Autodesk Inventor part; units mm, degrees
ref_plane "YZ Plane" through (0, 0, 0) normal (1, 0, 0) x (0, 1, 0)
ref_plane "XZ Plane" through (0, 0, 0) normal (0, 1, 0) x (-1, 0, 0)
ref_plane "XY Plane" through (0, 0, 0) normal (0, 0, 1) x (1, 0, 0)
sketch "Sketch1" plane through (0, 0, 0) normal (0, 1, 0) x (-1, 0, 0)
  line L0 (101.6, 101.6) -> (-101.6, 101.6)
  line L1 (-101.6, 101.6) -> (-101.6, -101.6)
  line L2 (-101.6, -101.6) -> (101.6, -101.6)
  line L3 (101.6, -101.6) -> (101.6, 101.6)
  circle A0 centre (0, 0) radius 2.5
  line L4 (9.525, -6.5) -> (-9.525, -6.5)
  line L5 (0, 0) -> (0, 8)
  line L6 (-14.5, -6.5) -> (-14.5, 22.5)
  line L7 (14.5, 22.5) -> (14.5, -6.5)
  circle A1 centre (0, 8) radius 14
  line L8 (-14.5, 22.5) -> (14.5, 22.5)
  line L9 (14.5, -6.5) -> (-14.5, -6.5)
  line L10 (-24.5, 32.5) -> (24.5, 32.5)
  line L11 (24.5, 32.5) -> (24.5, -16.5)
  line L12 (24.5, -16.5) -> (-24.5, -16.5)
  line L13 (-24.5, -16.5) -> (-24.5, 32.5)
  line L14 (-9.525, 22.5) -> (9.525, 22.5)
  line L15 (9.525, 22.5) -> (9.525, 27.58)
  line L16 (9.525, 27.58) -> (-9.525, 27.58)
  line L17 (-9.525, 27.58) -> (-9.525, 22.5)
  point P0 (9.525, 22.5)
  point P1 (-9.525, -6.5)
  dimension "d0" = 203.2
  dimension "d1" = 203.2
  dimension "d2" = 8
  dimension "d3" = 28
  dimension "d4" = 29
  dimension "d5" = 29
  dimension "d6" = 14.5
  dimension "d7" = 10
  dimension "d8" = 10
  dimension "d9" = 10
  dimension "d10" = 10
  dimension "d11" = 5.08
  dimension "d12" = 9.525
  dimension "d13" = 9.525
  dimension "d14" = 101.6
  dimension "d15" = 101.6
extrude "Extrusion1" add sketch "Sketch1" along normal blind 56.5 contours A0 | L4 L9 L6 L8 L7 | L8 L17 L16 L15 | A1 | L10 L11 L12 L13
sketch "Sketch2" plane through (0, 56.5, 0) normal (0, 1, 0) x (1, 0, 0)
  line L0 (101.6, 101.6) -> (-101.6, 101.6)
  line L1 (-101.6, 101.6) -> (-101.6, -101.6)
  line L2 (-101.6, -101.6) -> (101.6, -101.6)
  line L3 (101.6, -101.6) -> (101.6, 101.6)
  circle A0 centre (0, 0) radius 2.5
  line L4 (-9.525, 6.5) -> (9.525, 6.5)
  line L5 (0, 0) -> (0, -8)
  line L6 (14.5, 6.5) -> (14.5, -22.5)
  line L7 (-14.5, -22.5) -> (-14.5, 6.5)
  circle A1 centre (0, -8) radius 14
  line L8 (14.5, -22.5) -> (-14.5, -22.5)
  line L9 (-14.5, 6.5) -> (14.5, 6.5)
  line L10 (24.5, -32.5) -> (-24.5, -32.5)
  line L11 (-24.5, -32.5) -> (-24.5, 16.5)
  line L12 (-24.5, 16.5) -> (24.5, 16.5)
  line L13 (24.5, 16.5) -> (24.5, -32.5)
  line L14 (9.525, -22.5) -> (-9.525, -22.5)
  line L15 (-9.525, -22.5) -> (-9.525, -27.58)
  line L16 (-9.525, -27.58) -> (9.525, -27.58)
  line L17 (9.525, -27.58) -> (9.525, -22.5)
  point P0 (9.525, 22.5)
  point P1 (-9.525, -6.5)
  dimension "d18" = 203.2
  dimension "d19" = 203.2
  dimension "d20" = 8
  dimension "d21" = 28
  dimension "d22" = 29
  dimension "d23" = 29
  dimension "d24" = 14.5
  dimension "d25" = 10
  dimension "d26" = 10
  dimension "d27" = 10
  dimension "d28" = 10
  dimension "d29" = 5.08
  dimension "d30" = 9.525
  dimension "d31" = 9.525
  dimension "d32" = 101.6
  dimension "d33" = 101.6
extrude "Extrusion2" cut sketch "Sketch2" against normal blind 19.5 contours A0 | L4 L9 L6 L8 L7 | L8 L17 L16 L15 | A1
sketch "Sketch4" plane through (0, 56.5, 0) normal (0, 1, 0) x (1, 0, 0)
  circle A0 centre (-17.508, -8) radius 2
  circle A1 centre (17.4854, -8) radius 2
  circle A2 centre (17.4854, -8) radius 2
  circle A3 centre (0, -8.01) radius 14
  circle A4 centre (0, -0.01) radius 2.5
  circle A5 centre (-19.4934, 12.0285) radius 2.2448
  circle A6 centre (19.5, 12.0285) radius 2.3104
  circle A7 centre (19.5, -28.5182) radius 2.2008
  circle A8 centre (-19.4934, -28.5182) radius 2.3894
  point P0 (0, 0)
  dimension "d37" = 34.9934
  dimension "d38" = 28
  dimension "d39" = 8
  dimension "d65" = 8
  dimension "d66" = 8
hole "Hole1" at (-17.508, 56.5, 8) at (17.4854, 56.5, 8) at (-19.4934, 56.5, 28.5182) at (19.5, 56.5, 28.5182) at (-19.4934, 56.5, -12.0285) at (19.5, 56.5, -12.0285) direction (0, -1, 0) diameter 2.85 depth 12.7 tip angle 118 countersink diameter 3.0226 countersink angle 82
sketch "Sketch5" plane through (0, 0, 0) normal (0, -1, 0) x (1, 0, 0)
  circle A0 centre (-19.4934, 28.5182) radius 1.425
  circle A1 centre (-19.4934, 28.5182) radius 1.425
  circle A2 centre (19.5, 28.5182) radius 1.425
  circle A3 centre (19.5, 28.5182) radius 1.425
  circle A4 centre (19.5, -12.0285) radius 1.425
  circle A5 centre (19.5, -12.0285) radius 1.425
  circle A6 centre (-19.4934, -12.0285) radius 1.5113
  circle A7 centre (-19.4934, -12.0285) radius 1.5113
  point P0 (0, 0)
hole "Hole2" at (19.5, 0, -12.0285) at (-19.4934, 0, -12.0285) at (-19.4934, 0, 28.5182) at (19.5, 0, 28.5182) direction (0, 1, 0) diameter 2.85 depth 12.7 tip angle 118 countersink diameter 3.0226 countersink angle 82
sketch "Sketch6" plane through (-24.5, 0, 32.5) normal (0, 0, 1) x (1, 0, 0)
  line L0 (34.025, 56.5) -> (34.025, 37)
  line L1 (14.975, 56.5) -> (34.025, 56.5)
  line L2 (34.025, 56.5) -> (34.025, 46.75)
  line L3 (34.025, 46.75) -> (14.975, 46.75)
  line L4 (14.975, 46.75) -> (14.975, 56.5)
  point P0 (24.5, 0)
extrude "Extrusion3" cut sketch "Sketch6" against normal blind 25.4
sketch "Sketch8" plane through (0, 56.5, 0) normal (0, 1, 0) x (1, 0, 0)
  line L0 (-24.5, -3) -> (24.5, -3)
  line L1 (24.5, -3) -> (24.5, -13)
  line L2 (24.5, -13) -> (-24.5, -13)
  line L3 (-24.5, -13) -> (-24.5, -3)
  line L4 (14.5, 6.5) -> (14.5, -22.5)
  line L5 (14.5, -3) -> (14.5, -13)
  line L6 (-14.5, -22.5) -> (-14.5, 6.5)
  line L7 (-14.5, -3) -> (-14.5, -13)
  line L8 (24.5, -32.5) -> (24.5, 16.5)
  line L9 (-24.5, 16.5) -> (-24.5, -32.5)
  point P0 (0, 0)
  dimension "d58" = 10
  dimension "d60" = 0
  dimension "d61" = 0
  dimension "d62" = 3
extrude "Extrusion4" cut sketch "Sketch8" against normal blind 2 contours L0 L6 L2 L3 | L0 L1 L2 L4
sketch "Sketch9" plane through (0, 56.5, 0) normal (0, 1, 0) x (1, 0, 0)
  line L0 (-14.5, 6.5) -> (14.5, 6.5)
  line L1 (24.5, 16.5) -> (-24.5, 16.5)
  line L2 (-14.5, 6.5) -> (14.5, 6.5)
  line L3 (14.5, 6.5) -> (14.5, 16.5)
  line L4 (14.5, 16.5) -> (-14.5, 16.5)
  line L5 (-14.5, 16.5) -> (-14.5, 6.5)
  line L6 (14.5, 6.5) -> (14.5, -3)
  line L7 (-14.5, 11.5) -> (14.5, 11.5)
  line L8 (-24.5, 16.5) -> (-24.5, -32.5)
  line L9 (-14.5, 6.5) -> (-24.5, 6.5)
  line L10 (-24.5, 6.5) -> (-24.5, -22.5)
  line L11 (-24.5, -22.5) -> (-14.5, -22.5)
  line L12 (-14.5, -22.5) -> (-14.5, 6.5)
  line L13 (-9.525, -22.5) -> (-14.5, -22.5)
  line L14 (-20.5, 6.5) -> (-20.5, -22.5)
  line L15 (24.5, -32.5) -> (24.5, 16.5)
  line L16 (24.5, -22.5) -> (20.5, -22.5)
  line L17 (20.5, -22.5) -> (20.5, 6.5)
  line L18 (20.5, 6.5) -> (24.5, 6.5)
  line L19 (24.5, 6.5) -> (24.5, -22.5)
  point P0 (0, 0)
  point P1 (-14.5, 16.5)
  dimension "d67" = 0
  dimension "d68" = 5
  dimension "d69" = 0
  dimension "d71" = 4
  dimension "d72" = 4
extrude "Extrusion5" cut sketch "Sketch9" against normal through all contours L15 L16 L17 L18 | L5 L1 L3 L7 | L14 L11 L8 L9
sketch "Sketch11" plane through (0, 37, 0) normal (0, 1, 0) x (1, 0, 0)
  line L0 (-20.5, -3) -> (-14.5, -3)
  line L1 (20.5, -13) -> (20.5, -3)
  line L2 (-20.5, -3) -> (20.5, -3)
  line L3 (20.5, -3) -> (20.5, -13)
  line L4 (20.5, -13) -> (-20.5, -13)
  line L5 (-20.5, -13) -> (-20.5, -3)
  point P0 (0, 0)
  dimension "d75" = 41
  dimension "d76" = 10
sketch "Sketch12" plane through (14.5, 56.5, -11.5) normal (0, 0, -1) x (-1, 0, 0)
  line L0 (0, 0) -> (-6, 0)
  line L1 (29, 0) -> (29, -19.5)
  line L2 (0, 0) -> (29, 0)
  line L3 (29, 0) -> (29, -2)
  line L4 (29, -2) -> (0, -2)
  line L5 (0, -2) -> (0, 0)
  point P0 (14.5, -56.5)
  dimension "d77" = 2
extrude "Extrusion6" cut sketch "Sketch12" against normal blind 25.4
sketch "Sketch14" plane through (0, 56.5, 0) normal (0, 1, 0) x (1, 0, 0)
  line L0 (-14.5, 16.5) -> (-24.5, 16.5)
  line L1 (24.5, 6.5) -> (24.5, 16.5)
  line L2 (-24.5, 16.5) -> (24.5, 16.5)
  line L3 (24.5, 16.5) -> (24.5, 16)
  line L4 (24.5, 16) -> (-24.5, 16)
  line L5 (-24.5, 16) -> (-24.5, 16.5)
  line L6 (24.5, 16.5) -> (14.5, 16.5)
  line L7 (9.525, -32.5) -> (24.5, -32.5)
  line L8 (24.5, 16.5) -> (24, 16.5)
  line L9 (24, 16.5) -> (24, -32.5)
  line L10 (24, -32.5) -> (24.5, -32.5)
  line L11 (24.5, -32.5) -> (24.5, 16.5)
  line L12 (-24.5, -22.5) -> (-24.5, -32.5)
  line L13 (24.5, -32.5) -> (-24.5, -32.5)
  line L14 (-24.5, -32.5) -> (-24.5, -32)
  line L15 (-24.5, -32) -> (24.5, -32)
  line L16 (24.5, -32) -> (24.5, -32.5)
  line L17 (-24.5, -32.5) -> (-9.525, -32.5)
  line L18 (-24.5, -32.5) -> (-24, -32.5)
  line L19 (-24, -32.5) -> (-24, 16.5)
  line L20 (-24, 16.5) -> (-24.5, 16.5)
  line L21 (-24.5, 16.5) -> (-24.5, -32.5)
  point P0 (0, 0)
  point P1 (-24.5, 16)
  point P2 (24, 16)
  point P3 (24, -32)
  point P4 (-24, -32)
  point P5 (-24, 16)
  dimension "d89" = 0.5
  dimension "d90" = 0.5
  dimension "d91" = 0.5
  dimension "d92" = 0.5
extrude "Extrusion8" cut sketch "Sketch14" against normal through all contours L2 L9 L4 L19 L0 | L19 L4 L5 L0 | L19 L15 L12 L21 L4 | L2 L1 L4 L9 | L4 L1 L11 L15 L9 | L19 L13 L12 L15 | L15 L9 L7 L13 L19 | L15 L11 L7 L9
sketch "Sketch15" plane through (20.5, 56.5, 22.5) normal (1, 0, 0) x (0, 0, -1)
  point P0 (22.5, -56.5)
properties part number "Motor_Holder"
The listing builds one solid part. Answer for the finished solid, in the listing's coordinates (mm). A direction names the side the tool comes from. Coordinates: 2 decimals unless noted, no trailing zeros. Loops run counter-clockwise (first coordinate to the right, second up) from the corner with the lowest first, then second, coordinate; pieces in that order, holes last. Notation, with made-up numbers: (20.25, -3) -> (28.25, -3) arc R36 ccw to (28.25, 33) -> close; hole circle Ø1 at (89.25, -39.5). An arc over 180 degrees is marked (long way). Return JSON: item names as keys, results as strings. Group by question number.
(1) A cutting plane is placed at C-C on y = 4. Count the separate pieces of the cut face and the enclosed holes in it, and give its area (3 significant figures).
(2) A cutting plane is placed at D-D on y = 16. Write down the section's boundary in (x, z).
(3) A cutting plane is placed at B-B on x = -6.5. Write down the section's boundary in (y, z).
(4) Which of the six approach directions +Z, -Z, +X, -X, +Y, -Y give full straight-line access (tool end or side, diameter ignored) to faces 1 (the cylindrical face through (20.89, 50.01, 28.21)), 2 (the cylindrical face through (20.89, 6.49, -11.72)), 3 (the flat face through (17, 56, 3)), 4 (the flat face through (22, 29, 22.5))?
(5) Determine the mould class of faces 5 (the flat face through (0, 0, 8)), 6 (the conical face through (-17.75, 43.09, 7.95)) for opening direction Z: released by +Z, released by -Z, zero draft, split by the parting line, or undercut.
(6) A cutting plane is placed at A-A on z = -0.5. Write down the section's boundary in (x, y), and give its area (3 significant figures).
(7) Find the intervals of material crossed by probe 1 along X at (y, z) = (46.5, 8); probe 2 along Z at (x, y) = (19, 5); probe 3 along X at (y, z) = (51.5, -4.5), in increasing order. Write a range as from..to.
(8) Given pin 1 Ø5 at (x, z) = (18, 7) entering from +Y; pin 2 Ø5 at (x, y) = (-5.5, 42) entering from -Z; pin 3 Ø5 at (y, z) = (39, 6.5) entering from +X, each flat-ended and moving along its own axis, determine where each tip first touches the part or whether it passes through.
The answers:
{
 "1": {"separate pieces": "1", "enclosed holes": "4", "area": "1,940 mm^2"},
 "2": {"outline": "(-24, -16) -> (-14.5, -16) -> (-14.5, -11.5) -> (14.5, -11.5) -> (14.5, -16) -> (24, -16) -> (24, -6.5) -> (20.5, -6.5) -> (20.5, 22.5) -> (24, 22.5) -> (24, 32) -> (-24, 32) -> (-24, 22.5) -> (-20.5, 22.5) -> (-20.5, -6.5) -> (-24, -6.5) -> close"},
 "3": {"outline": "(0, -11.5) -> (54.5, -11.5) -> (54.5, -6.5) -> (37, -6.5) -> (37, 27.58) -> (46.75, 27.58) -> (46.75, 32) -> (0, 32) -> close"},
 "4": {"face 1": "+Y", "face 2": "-Y", "face 3": "+X, -X, +Y", "face 4": "+X, +Y, -Y"},
 "5": {"face 5": "zero draft", "face 6": "undercut"},
 "6": {"outline": "(-20.5, 0) -> (20.5, 0) -> (20.5, 56.5) -> (14.5, 56.5) -> (14.5, 37) -> (-14.5, 37) -> (-14.5, 56.5) -> (-20.5, 56.5) -> close", "area": "1,750 mm^2"},
 "7": {"probe 1": "x = -20.5..-18.93, -16.08..-14.5, 14.5..16.06, 18.91..20.5", "probe 2": "z = -16..-13.36, -10.69..27.18, 29.85..32", "probe 3": "x = -20.5..-14.5, 14.5..20.5"},
 "8": {"pin 1": "stops at y = 54.5", "pin 2": "stops at z = -11.5", "pin 3": "stops at x = 20.5"}
}
